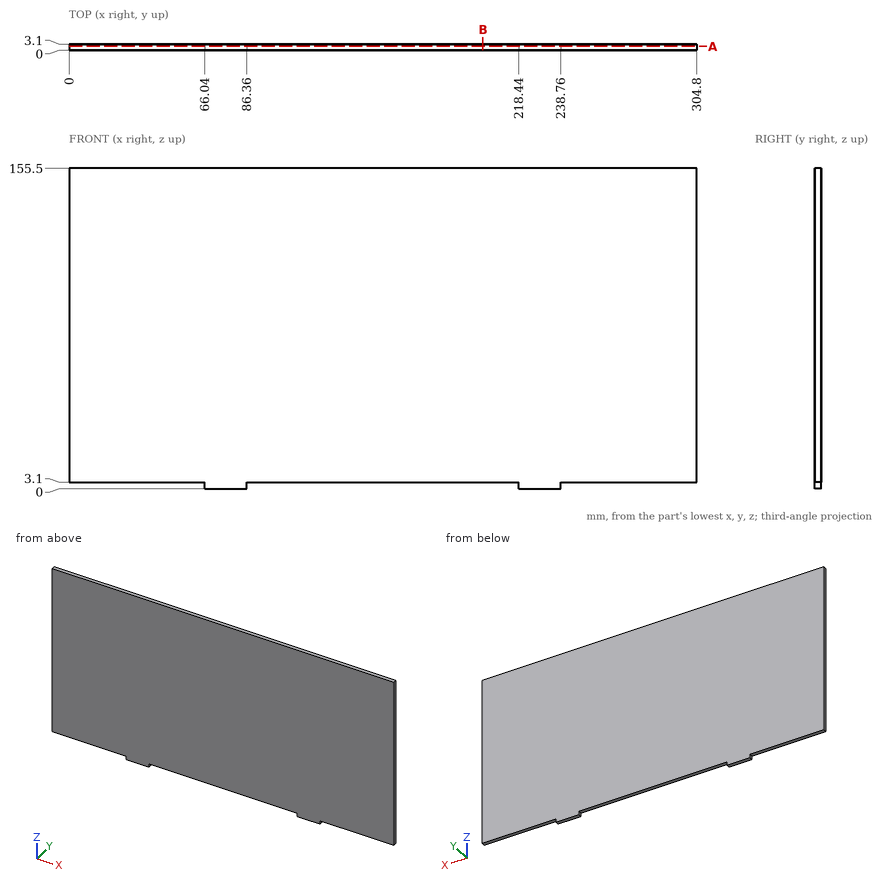
The drawing under review shows one solid part. Ordinate dimensions are in mm from its lowest x, y, z. Coordinates: 2 decimals unless noted, no trailing zeros. Write each loop counter-clockwise with the first axis right and the second up, starting at its lowest first coordinate (ties: lowest second). Pieces come first, ordered by that corner, then holes.
1) Add section A-A (y = 1.95). Write out the cut boundary in (x, z), plus the area to 3 significant figures.
2) To check wall thickness, follow L1, parallel to Z at x = 145.5, y = 1.7. State the ranges of the line that lie inside material, in increasing order.
3) Insertion check: pin 1 (0.9 mm diameter, centred on x = 281, y = 1, fed in from -Z); pin 2 (0.9 mm diameter, centred on y = 1.5, z = 1, fed in from +X). Each pin has a flat end and moves straight along its axis. Give the tip position at first contact, or say it passes through.
4) Add section B-B (x = 201). Write out the cut boundary in (y, z).
Check result:
1. outline: (0, 3.1) - (66.04, 3.1) - (66.04, 0) - (86.36, 0) - (86.36, 3.1) - (218.44, 3.1) - (218.44, 0) - (238.76, 0) - (238.76, 3.1) - (304.8, 3.1) - (304.8, 155.5) - (0, 155.5) - close
1. area: 46,600 mm2
2. L1: z = 3.1 to 155.5
3. pin 1: stops at z = 3.1
3. pin 2: stops at x = 238.76
4. outline: (0, 3.1) - (3.1, 3.1) - (3.1, 155.5) - (0, 155.5) - close
